Part model, mm, in its own coordinate system. Face numbers are marked on the shaded views. Coordinates: 2 decimals unless noted, no trailing zeros. Use a Markdown table: item, result. Add a question column.
1) Wall check: L1, parallel to X at y = 15, z = -26.5; L2, parallel to Y at x = 1048.5, z = -12; L3, parallel to X at y = 255, z = -36.5. Give the ranges that are in metal, low to high. Write a range as [from, to].
2) Two-plate mould, pull along Y, no slides. Class the marked faces 1, 2 and 3: +Y half, -Y half, draft (parallel to the pull), parting line (faces both ways), or undercut.
3) Drop flat-ended pins along their axis: P1, Ø2, axis at y = 68, z = -17, coming from the +X side; P2, Ø12.5, axis at x = 1055, y = 248.5, coming from the -Z side; P3, Ø3, axis at x = 1530, y = 180.5, coming from the -Z side; P4, Ø1, axis at x = 1092, y = 185.5, coming from the -Z side. Give the stop position or say it passes through.
```python
from build123d import *

# Parameters (mm, degrees)
SKETCH2_W                    = 1066.8
SKETCH2_H                    = 304.8
BOSS_EXTRUDE1_DEPTH          = 50.8
CUT_EXTRUDE1_DEPTH           = 1107.294920223
CUT_EXTRUDE1_DEPTH_BACK      = 1107.294920223
SKETCH4_R                    = 7.14375
CUT_EXTRUDE3_DEPTH           = 1037.520325732
FILLET4_R                    = 6.35
REGISTRATION_HOLE_SKETCH_R   = 12.7
BASE_REGISTRATION_HOLE_DEPTH = 50.8
LPATTERN3_COUNT              = 4
LPATTERN3_PITCH              = 304.8
LPATTERN3_COUNT_DIR2         = 2
LPATTERN3_PITCH_DIR2         = 228.6
SKETCH7_R                    = 76.2
CUT_EXTRUDE4_DEPTH           = 12.7
FILLET5_R                    = 12.7


# Read off the part's stored shape, not the designer's step: Indent1
with BuildPart() as part:
    # Sketch2 → Boss-Extrude1 (new, symmetric)
    with BuildSketch(Plane.XY):
        with Locations((1206.465176028, 136.123084384)):
            Rectangle(SKETCH2_W, SKETCH2_H)
    extrude(amount=BOSS_EXTRUDE1_DEPTH, both=True)

    # Indent1 outline → Indent1 (revolve, cut)
    with BuildSketch(Plane(origin=(0, 136.123084384, -50.8), x_dir=(0, 1, 0), z_dir=(0, 0, -1))):
        with BuildLine():
            Line((76.2, 1667.322776028), (0, 1667.322776028))
            Line((0, 1667.322776028), (0, 745.607576028))
            Line((0, 745.607576028), (23.064945381, 745.607576028))
            add(Edge.make_bspline(
                [(23.064945381, 745.607576028), (23.566825523, 748.91437787), (25.363204219, 760.90488429), (28.330664868, 781.598898763), (31.871058885, 807.703400336), (35.241099853, 833.832092117), (38.460845457, 859.980959498), (42.572514827, 894.869141414), (47.400937928, 938.517112788), (52.760650205, 990.942462001), (57.722301111, 1043.408031291), (62.308317352, 1095.908289185), (67.933123727, 1165.949858053), (72.828043506, 1236.047318759), (76.911244662, 1306.192759412), (79.080505646, 1350.052513699), (80.485669281, 1383.896744518), (81.068244998, 1400.195093482), (81.313954963, 1407.717593946)],
                knots=[0.116308657, 0.116308657, 0.116308657, 0.116308657, 0.125901739, 0.151082086, 0.176262434, 0.201442782, 0.22662313, 0.251803477, 0.302164173, 0.352524868, 0.402885564, 0.453246259, 0.503606955, 0.604328346, 0.654689041, 0.705049737, 0.730230084, 0.75181382, 0.75181382, 0.75181382, 0.75181382], degree=3))
            ThreePointArc((81.313954963, 1407.717593946), (80.564993874, 1410.923022844), (78.31179575, 1413.322776028))
            ThreePointArc((78.31179575, 1413.322776028), (76.063072477, 1415.714189378), (75.309046779, 1418.909038266))
            add(Edge.make_bspline(
                [(75.309046779, 1418.909038266), (75.323959024, 1419.411481069), (75.408519742, 1422.276130669), (75.558482998, 1427.503133809), (75.676289458, 1432.228116929), (75.735192688, 1434.590608489), (75.838475179, 1438.733064052), (76.045040161, 1447.017975177), (76.2, 1459.45016933), (76.2, 1467.737655163), (76.2, 1471.88139808), (76.2, 1476.663773407), (76.2, 1486.228524062), (76.2, 1500.575650045), (76.2, 1510.1404007), (76.2, 1514.922776028), (76.2, 1565.722776028), (76.2, 1616.522776028), (76.2, 1667.322776028)],
                knots=[0.761574077, 0.761574077, 0.761574077, 0.761574077, 0.763021384, 0.769825774, 0.776630163, 0.776630163, 0.776630163, 0.788561161, 0.800492159, 0.812423157, 0.812423157, 0.812423157, 0.826192956, 0.839962756, 0.853732555, 0.853732555, 0.853732555, 1, 1, 1, 1], degree=3))
        make_face()
    revolve(axis=Axis((0, 136.123084384, -50.8), (1, 0, 0)), mode=Mode.SUBTRACT)

    # Sketch4 → Cut-Extrude1 (cut, two sides: drawn at the far end of the back side and taken through both)
    with BuildSketch(Plane.ZY.offset(-1739.865176028).offset(-CUT_EXTRUDE1_DEPTH_BACK)):
        with Locations((-50.8, 136.123084384)):
            Circle(SKETCH4_R)
    extrude(amount=CUT_EXTRUDE1_DEPTH + CUT_EXTRUDE1_DEPTH_BACK, mode=Mode.SUBTRACT)

    # Sketch6 → Cut-Extrude3 (cut, through all)
    with BuildSketch(Plane.ZY.offset(-1667.322776028)):
        with BuildLine():
            Line((22.980332745, 117.073084384), (-50.8, 117.073084384))
            Line((-50.8, 117.073084384), (-50.8, 59.923084384))
            ThreePointArc((-50.8, 59.923084384), (-4.1372204, 75.881694958), (22.980332745, 117.073084384))
        make_face()
        with BuildLine():
            Line((-50.8, 155.173084384), (22.980332745, 155.173084384))
            ThreePointArc((22.980332745, 155.173084384), (-4.1372204, 196.364473811), (-50.8, 212.323084384))
            Line((-50.8, 212.323084384), (-50.8, 199.623084384))
            Line((-50.8, 199.623084384), (-50.8, 155.173084384))
        make_face()
    extrude(amount=-CUT_EXTRUDE3_DEPTH, mode=Mode.SUBTRACT)

    # Fillet4
    fillet4_edges = [part.edges().sort_by_distance(p)[0] for p in [
        (745.607576028, 136.123084384, -27.735054619),
    ]]
    fillet(fillet4_edges, radius=FILLET4_R)

    # Registration Hole Sketch → Base-Registration-Hole (cut)
    with BuildSketch(Plane(origin=(0, 0, -50.8), x_dir=(-1, 0, 0), z_dir=(0, 0, -1))):
        with Locations((-745.607576028, 21.823084384)):
            Circle(REGISTRATION_HOLE_SKETCH_R)
    base_registration_hole = extrude(amount=-BASE_REGISTRATION_HOLE_DEPTH, mode=Mode.SUBTRACT)

    # LPattern3: Base-Registration-Hole 4 × 2
    with Locations(*[(i * LPATTERN3_PITCH, j * LPATTERN3_PITCH_DIR2, 0) for i in range(LPATTERN3_COUNT) for j in range(LPATTERN3_COUNT_DIR2) if (i, j) != (0, 0)]):
        add(base_registration_hole, mode=Mode.SUBTRACT)

    # Sketch7 → Cut-Extrude4 (cut)
    with BuildSketch(Plane.ZY.offset(-1667.322776028)):
        with Locations((-50.8, 136.123084384)):
            Circle(SKETCH7_R)
    extrude(amount=-CUT_EXTRUDE4_DEPTH, mode=Mode.SUBTRACT)

    # Fillet5
    # the kernel refuses this fillet: 12.7 mm, written as the material it adds along each edge
    with BuildSketch(Plane(origin=(1680.022776028, 136.123084384, -50.8), x_dir=(0, -0.6204773534699832, 0.7842243644716003), z_dir=(0, -0.7842243644716003, -0.6204773534699832))) as fillet5_piece_1_section:
        with BuildLine():
            CenterArc((76.2 - FILLET5_R, FILLET5_R), FILLET5_R, 270, 90)
            Line((76.2 - FILLET5_R, 0), (76.2, 0))
            Line((76.2, 0), (76.2, FILLET5_R))
        make_face()
    fillet5_piece_1 = revolve(axis=Axis((1680.022776028, 136.123084384, -50.8), (-1, 0, 0)), revolution_arc=38.351001738, mode=Mode.PRIVATE)
    fillet5_piece_1 = split(fillet5_piece_1, bisect_by=Plane(origin=(1677.149054572, 117.073084384, 21.679553224), z_dir=(0, 1, 0)), keep=Keep.TOP, mode=Mode.PRIVATE)
    add(fillet5_piece_1)
    with BuildSketch(Plane(origin=(1680.022776028, 117.073084384, 22.980332745), x_dir=(0, -0.9256147934109615, -0.37846697903355186), z_dir=(1, 0, 0))) as fillet5_piece_2:
        with BuildLine():
            CenterArc((18.865839358, 12.583660567), FILLET5_R, 157.761243907, 120)
            Line((7.110531482, 17.390191201), (0, 0))
            ThreePointArc((0, 0), (10.290457832, -0.698036598), (20.580915663, 0))
        make_face()
    extrude(amount=59.8424)
    with BuildSketch(Plane(origin=(1680.022776028, 155.173084384, 22.980332745), x_dir=(0, 0, -1), z_dir=(1, 0, 0))) as fillet5_piece_3:
        with BuildLine():
            CenterArc((18.787719605, 12.7), FILLET5_R, 150, 120)
            ThreePointArc((7.789196977, 19.05), (3.248485487, 9.789183802), (0, 0))
            Line((0, 0), (18.787719605, 0))
        make_face()
    extrude(amount=59.8424)
    with BuildSketch(Plane(origin=(1680.022776028, 136.123084384, -50.8), x_dir=(0, 0, 1), z_dir=(0, -1, 0))) as fillet5_piece_4_section:
        with BuildLine():
            CenterArc((76.2 - FILLET5_R, FILLET5_R), FILLET5_R, 270, 90)
            Line((76.2, FILLET5_R), (76.2, 0))
            Line((76.2, 0), (76.2 - FILLET5_R, 0))
        make_face()
    fillet5_piece_4 = revolve(axis=Axis((1680.022776028, 136.123084384, -50.8), (-1, 0, 0)), revolution_arc=38.351001738, mode=Mode.PRIVATE)
    fillet5_piece_4 = split(fillet5_piece_4, bisect_by=Plane(origin=(1677.14905497, 155.173084384, 21.679553319), z_dir=(0, -1, 0)), keep=Keep.TOP, mode=Mode.PRIVATE)
    add(fillet5_piece_4)
    with BuildSketch(Plane(origin=(1628.570486869, 117.073084384, 22.980332745), x_dir=(0, -0.9256147934109611, -0.378466979033553), z_dir=(1, 0, 0))) as fillet5_piece_5a_section:
        with BuildLine():
            CenterArc((18.865839358, 12.583660567), FILLET5_R, 157.761243907, 120)
            Line((7.110531482, 17.390191201), (0, 0))
            ThreePointArc((0, 0), (10.290457832, -0.698036598), (20.580915663, 0))
        make_face()
    fillet5_piece_5a = extrude(amount=111.294689159, mode=Mode.PRIVATE)
    fillet5_piece_5a = split(fillet5_piece_5a, bisect_by=Plane(origin=(1680.022776028, 112.40455017, 17.056705553), z_dir=(-1, 0, 0)), keep=Keep.TOP, mode=Mode.PRIVATE)
    with BuildSketch(Plane(origin=(1680.022776028, 136.123084384, -50.8), x_dir=(0, -0.6204773534699832, 0.7842243644716003), z_dir=(0, -0.7842243644716003, -0.6204773534699832))) as fillet5_piece_5b_section:
        with BuildLine():
            CenterArc((76.2 - FILLET5_R, FILLET5_R), FILLET5_R, 270, 90)
            Line((76.2 - FILLET5_R, 0), (76.2, 0))
            Line((76.2, 0), (76.2, FILLET5_R))
        make_face()
    fillet5_piece_5b = revolve(axis=Axis((1680.022776028, 136.123084384, -50.8), (-1, 0, 0)), revolution_arc=38.351001738, mode=Mode.PRIVATE)
    fillet5_piece_5b = split(fillet5_piece_5b, bisect_by=Plane(origin=(1677.047146673, 117.073084384, 14.411791174), z_dir=(0, -1, 0)), keep=Keep.TOP, mode=Mode.PRIVATE)
    fillet5_piece_5 = fillet5_piece_5a & fillet5_piece_5b
    add(fillet5_piece_5)
    with BuildSketch(Plane(origin=(1680.022776028, 136.123084384, -50.8), x_dir=(0, 0, 1), z_dir=(0, -1, 0))) as fillet5_piece_6a_section:
        with BuildLine():
            CenterArc((76.2 - FILLET5_R, FILLET5_R), FILLET5_R, 270, 90)
            Line((76.2, FILLET5_R), (76.2, 0))
            Line((76.2, 0), (76.2 - FILLET5_R, 0))
        make_face()
    fillet5_piece_6a = revolve(axis=Axis((1680.022776028, 136.123084384, -50.8), (-1, 0, 0)), revolution_arc=38.351001738, mode=Mode.PRIVATE)
    fillet5_piece_6a = split(fillet5_piece_6a, bisect_by=Plane(origin=(1677.047146631, 155.173084384, 14.41179131), z_dir=(0, 1, 0)), keep=Keep.TOP, mode=Mode.PRIVATE)
    with BuildSketch(Plane(origin=(1628.570486869, 155.173084384, 22.980332745), x_dir=(0, 0, -1), z_dir=(1, 0, 0))) as fillet5_piece_6b_section:
        with BuildLine():
            CenterArc((18.787719605, 12.7), FILLET5_R, 150, 120)
            ThreePointArc((7.789196977, 19.05), (3.248485487, 9.789183802), (0, 0))
            Line((0, 0), (18.787719605, 0))
        make_face()
    fillet5_piece_6b = extrude(amount=111.294689159, mode=Mode.PRIVATE)
    fillet5_piece_6b = split(fillet5_piece_6b, bisect_by=Plane(origin=(1680.022776028, 159.841618598, 17.056705553), z_dir=(-1, 0, 0)), keep=Keep.TOP, mode=Mode.PRIVATE)
    fillet5_piece_6 = fillet5_piece_6a & fillet5_piece_6b
    add(fillet5_piece_6)


solid = part.part
```
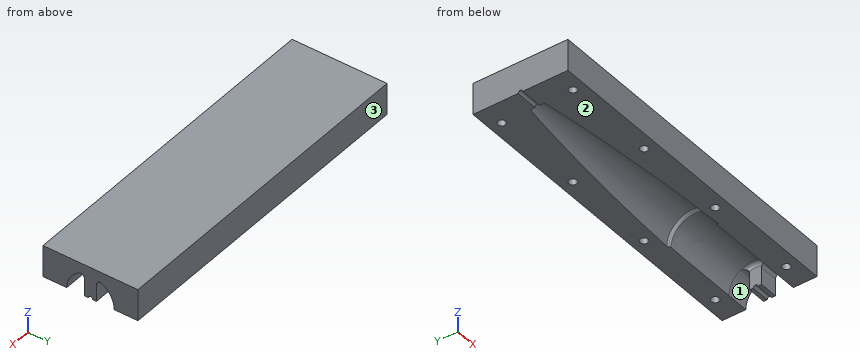
Results are:
| question | item | result |
|---|---|---|
| 1 | L1 | [673.07, 734.9], [756.32, 1039.7], [1061.12, 1344.5], [1365.92, 1649.3], [1670.72, 1739.87] |
| 1 | L2 | [-16.28, 9.27], [34.38, 92.85], [179.4, 237.87], [262.98, 288.52] |
| 1 | L3 | [673.07, 733.76], [757.45, 1038.56], [1062.25, 1343.36], [1367.05, 1648.16], [1671.85, 1739.87] |
| 2 | face 1 | undercut |
| 2 | face 2 | draft |
| 2 | face 3 | +Y half |
| 3 | P1 | x = 1739.87 |
| 3 | P2 | z = 0 |
| 3 | P3 | z = 10.04 |
| 3 | P4 | z = -14.11 |
